Could you check a few things on this model? Use its own coordinates, in mm. Give positions to 0.01 mm unless a question says otherwise; leave off trailing zeros. Loops run counter-clockwise (first coordinate to the right, second up) from the corner with the lowest first, then second, coordinate; pieces in that order, holes last. Notation, with made-up numbers: (13.25, 71.25) - (49.25, 71.25) arc R21 cw to (49.25, 76.25) - close; hole circle Ø8 at (43.5, 49.25). An arc over 180 degrees is marked (long way). Write each question's results on one line, items separated by ' | '. Start each with the question number.
1) I want a section at B-B, the plane y = -18.5. Write out the boundary of the cut face in (x, z), and give its area (3 significant figures).
2) I want a section at A-A, the plane y = -8. Write out the boundary of the cut face in (x, z), and give its area (3 significant figures).
3) I'm going to push flat-ended pins straight in: pin 1 (7.5 mm diameter, centred on x = -36, y = 10, fed in from +Z); pin 2 (1 mm diameter, centred on y = -9, z = 1, fed in from -X); pin 3 (1.5 mm diameter, centred on y = -13.5, z = 1, fed in from +X); pin 4 (6 mm diameter, centred on x = -31, y = -8, fed in from +Z). Where does each tip first touch, or does it pass through?
4) If I drill on probe 1 along Y at (x, z) = (0, 1.45); probe 2 along Y at (x, z) = (61, 0.2); probe 3 along Z at (x, y) = (55, 2.5), over which ranges is the centre line in solid material (lowest first)? Write a range as [from, to].
from build123d import *

# Parameters (mm, degrees)
F0_W      = 97.5
F0_H      = 15
F1_DEPTH  = 1
F2_W      = 77.5
F2_H      = 2.5
F3_DEPTH  = 3.5
F4_DEPTH  = 3.5
F5_R      = 10
F7_DEPTH  = 3.5
F10_DEPTH = 3.5


# Not quite as in the source:
# - a feature of the source that left no trace in its solid (it failed there, or was rolled back) is left out
# - a feature names something its author has since deleted; it is built from what else it names


with BuildPart() as f1:
    # F0 (on Top) → F1 (new body)
    with BuildSketch(Plane.XY):
        with Locations((-48.75, 7.5)):
            Rectangle(F0_W, F0_H)
        with Locations((48.75, 7.5)):
            Rectangle(F0_W, F0_H)
    extrude(amount=F1_DEPTH)

    # F2 (on Top) → F3 (join)
    with BuildSketch(Plane.XY):
        with Locations((58.75, -1.25)):
            Rectangle(F2_W, F2_H)
        with Locations((-58.75, -1.25)):
            Rectangle(F2_W, F2_H)
        with BuildLine():
            ThreePointArc((-17.3205080757, -2.5), (-16.5138781887, -1.2176320229), (-15.612494996, 0))
            Line((-15.612494996, 0), (-20, 0))
            Line((-20, 0), (-20, -2.5))
            Line((-20, -2.5), (-17.3205080757, -2.5))
        make_face()
        with BuildLine():
            ThreePointArc((-20, -12.5), (-19.3185165258, -7.3236190979), (-17.3205080757, -2.5))
            Line((-17.3205080757, -2.5), (-20, -2.5))
            Line((-20, -2.5), (-20, -12.5))
        make_face()
        with BuildLine():
            Line((20, 0), (15.612494996, 0))
            ThreePointArc((15.612494996, 0), (16.5138781887, -1.2176320229), (17.3205080757, -2.5))
            Line((17.3205080757, -2.5), (20, -2.5))
            Line((20, -2.5), (20, 0))
        make_face()
        with BuildLine():
            Line((20, -2.5), (17.3205080757, -2.5))
            ThreePointArc((17.3205080757, -2.5), (19.3185165258, -7.3236190979), (20, -12.5))
            Line((20, -12.5), (20, -2.5))
        make_face()
    extrude(amount=F3_DEPTH)

    # F2 (on Top) → F4 (join)
    with BuildSketch(Plane.XY):
        with BuildLine():
            Line((15.612494996, 0), (0, 0))
            Line((0, 0), (-15.612494996, 0))
            ThreePointArc((-15.612494996, 0), (-16.5138781887, -1.2176320229), (-17.3205080757, -2.5))
            Line((-17.3205080757, -2.5), (17.3205080757, -2.5))
            ThreePointArc((17.3205080757, -2.5), (16.5138781887, -1.2176320229), (15.612494996, 0))
        make_face()
        with BuildLine():
            ThreePointArc((20, -12.5), (19.3185165258, -7.3236190979), (17.3205080757, -2.5))
            Line((17.3205080757, -2.5), (-17.3205080757, -2.5))
            ThreePointArc((-17.3205080757, -2.5), (-19.3185165258, -7.3236190979), (-20, -12.5))
            Line((-20, -12.5), (20, -12.5))
        make_face()
        with BuildLine():
            ThreePointArc((-20, -12.5), (0, -32.5), (20, -12.5))
            Line((20, -12.5), (-20, -12.5))
        make_face()
    extrude(amount=F4_DEPTH)

    # F6: union 

    # F5 (on face) → F7 (cut)
    with BuildSketch(Plane.XY.offset(3.5)):
        with Locations((0, -12.5)):
            Circle(F5_R)
    extrude(amount=-F7_DEPTH, mode=Mode.SUBTRACT)

    # F8 (on face) → F10 (join)
    with BuildSketch(Plane.XY.offset(3.5)):
        with BuildLine():
            add(Edge.make_bspline(
                [(-97.5, 2.5), (-65, 1.25), (-32.5, 0), (0, 0)],
                knots=[0, 0, 0, 0, 0.5, 0.5, 0.5, 0.5], degree=3))
            Line((-97.5, 2.5), (-97.5, 0))
            Line((-97.5, 0), (0, 0))
        make_face()
        with BuildLine():
            add(Edge.make_bspline(
                [(0, 0), (32.5, 0), (65, 1.25), (97.5, 2.5)],
                knots=[0.5, 0.5, 0.5, 0.5, 1, 1, 1, 1], degree=3))
            Line((0, 0), (97.5, 0))
            Line((97.5, 0), (97.5, 2.5))
        make_face()
    extrude(amount=-F10_DEPTH)


solid = f1.part
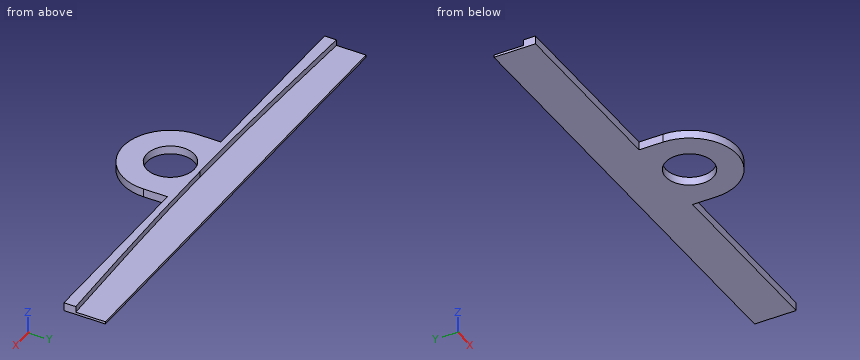
Answers:
1) outline: (-19.08, 0) - (-8, 0) - (-8, 3.5) - (-19.08, 3.5) - close; (8, 0) - (19.08, 0) - (19.08, 3.5) - (8, 3.5) - close | area: 77.6 mm2
2) outline: (-20, 0) - (-8.93, 0) - (-8.93, 3.5) - (-20, 3.5) - close; (8.93, 0) - (20, 0) - (20, 3.5) - (8.93, 3.5) - close | area: 77.5 mm2
3) pin 1: stops at z = 1 | pin 2: stops at x = -20 | pin 3: stops at x = 20 | pin 4: passes through
4) probe 1: y = [-32.5, -22.5], [-2.5, 0] | probe 2: y = [-2.5, 15] | probe 3: z = [0, 1]
